```python
from build123d import *

# Parameters (mm, degrees)
SKETCH_1_W      = 44
SKETCH_1_H      = 3
SKETCH_1_H_2    = 10
EXTRUDE_1_DEPTH = 4
SKETCH_1_3_W    = 44
SKETCH_1_3_H    = 3
EXTRUDE_2_DEPTH = 30
FILLET_1_R      = 1


with BuildPart() as part:
    # Sketch 1 → Extrude 1 (new body)
    with BuildSketch(Plane.XY):
        with BuildLine():
            ThreePointArc((-22, 1), (-21.707106781, 0.292893219), (-21, 0))
            Line((-21, 0), (21, 0))
            ThreePointArc((21, 0), (21.707106781, 0.292893219), (22, 1))
            Line((22, 1), (22, 104))
            Line((22, 104), (-22, 104))
            Line((-22, 104), (-22, 1))
        make_face()
        with BuildLine():
            ThreePointArc((3.25, 7), (0, 3.75), (-3.25, 7))
            Line((-3.25, 7), (-3.25, 57))
            ThreePointArc((-3.25, 57), (0, 60.25), (3.25, 57))
            Line((3.25, 57), (3.25, 7))
        make_face(mode=Mode.SUBTRACT)
        with BuildLine():
            ThreePointArc((-15.25, 97), (-12, 100.25), (-8.75, 97))
            Line((-8.75, 97), (-8.75, 47))
            ThreePointArc((-8.75, 47), (-12, 43.75), (-15.25, 47))
            Line((-15.25, 47), (-15.25, 97))
        make_face(mode=Mode.SUBTRACT)
        with BuildLine():
            Line((8.75, 47), (8.75, 97))
            ThreePointArc((8.75, 97), (12, 100.25), (15.25, 97))
            Line((15.25, 97), (15.25, 47))
            ThreePointArc((15.25, 47), (12, 43.75), (8.75, 47))
        make_face(mode=Mode.SUBTRACT)
        with Locations((0, 105.5)):
            Rectangle(SKETCH_1_W, SKETCH_1_H)
        with Locations((0, 112)):
            Rectangle(SKETCH_1_W, SKETCH_1_H_2)
        with BuildLine():
            Line((-22, 120), (-22, 117))
            Line((-22, 117), (22, 117))
            Line((22, 117), (22, 120))
            ThreePointArc((22, 120), (21.707106781, 120.707106781), (21, 121))
            Line((21, 121), (-21, 121))
            ThreePointArc((-21, 121), (-21.707106781, 120.707106781), (-22, 120))
        make_face()
    extrude(amount=EXTRUDE_1_DEPTH)

    # Sketch 1_3 → Extrude 2 (add)
    with BuildSketch(Plane.XY):
        with Locations((0, 105.5)):
            Rectangle(SKETCH_1_3_W, SKETCH_1_3_H)
        with BuildLine():
            Line((-22, 120), (-22, 117))
            Line((-22, 117), (22, 117))
            Line((22, 117), (22, 120))
            ThreePointArc((22, 120), (21.707106781, 120.707106781), (21, 121))
            Line((21, 121), (-21, 121))
            ThreePointArc((-21, 121), (-21.707106781, 120.707106781), (-22, 120))
        make_face()
    extrude(amount=-EXTRUDE_2_DEPTH)

    # Fillet 1
    fillet_1_edges = [part.edges().sort_by_distance(p)[0] for p in [
        (-22, 105.5, -30),
        (22, 105.5, -30),
        (0, 104, -30),
        (0, 107, -30),
        (0, 121, -30),
        (21.707106781, 120.707106781, -30),
        (22, 118.5, -30),
        (0, 117, -30),
        (-22, 118.5, -30),
        (-21.707106781, 120.707106781, -30),
    ]]
    fillet(fillet_1_edges, radius=FILLET_1_R)


solid = part.part
```
The model under review builds one solid part; all positions refer to its coordinate system, in mm. A direction names the side the tool comes from. Round coordinates to 2 decimals unless told otherwise and drop trailing zeros. Loops run counter-clockwise (first coordinate to the right, second up) from the corner with the lowest first, then second, coordinate; pieces in that order, holes last. Notation, with made-up numbers: M 78.25,-2.5 L 131.25,-2.5 A17 cw 131.25,30.5 Z; hole C 3.5,87.25 d6. An arc over 180 degrees is marked long. Write item = value, one per line.
Item 1: The part is to be moulded in two halves that separate along X. For faces 1 (the cylindrical face through (0.07, 3.75, 1.97)), 2 (the cylindrical face through (-12.07, 100.25, 1.97)), 3 (the flat face through (-22, 78, 2)), 4 (the flat face through (0, 112, 0)), say which applies: released by +X, released by -X, zero draft, split by the parting line, or undercut.
Return value:
face_1 = undercut
face_2 = undercut
face_3 = released by -X
face_4 = zero draft
Item 2: Insertion check: P1, Ø13, axis at x = -0.5, y = 31, coming from the -Z side; P2, Ø4, axis at x = -4, z = -24, coming from the -Y side. Each pin has a flat end and moves straight along its axis. Give the tip position at first contact, or say it passes through.
Return value:
P1 = 0
P2 = 104
Item 3: Take a section at A-A on z = -27. Write out the cut boundary in (x, y).
Return value:
outline = M -22,104 L 22,104 L 22,107 L -22,107 Z; M -22,117 L 22,117 L 22,120 A1 ccw 21,121 L -21,121 A1 ccw -22,120 Z
Item 4: Take a section at B-B on y = 52.5. Write out the cut boundary in (x, z), then the cut area to 3 significant figures.
Return value:
outline = M -22,0 L -15.25,0 L -15.25,4 L -22,4 Z; M -8.75,0 L -3.25,0 L -3.25,4 L -8.75,4 Z; M 3.25,0 L 8.75,0 L 8.75,4 L 3.25,4 Z; M 15.25,0 L 22,0 L 22,4 L 15.25,4 Z
area = 98.0 mm2
Item 5: Take a section at C-C on x = 0. Write out the cut boundary in (y, z), then the cut area to 3 significant figures.
Return value:
outline = M 0,0 L 3.75,0 L 3.75,4 L 0,4 Z; M 60.25,0 L 104,0 L 104,-29 A1 ccw 105,-30 L 106,-30 A1 ccw 107,-29 L 107,0 L 117,0 L 117,-29 A1 ccw 118,-30 L 120,-30 A1 ccw 121,-29 L 121,4 L 60.25,4 Z
area = 467 mm2
Item 6: For line 1 (Y direction, x = 13, z = -22.5); line 2 (Z direction, x = -5.5, y = 22), list the stretches that pass through material, from the lowest coordinate up. Write a range as [from, to].
Return value:
line_1 = [104, 107], [117, 121]
line_2 = [0, 4]
Item 7: Take a section at D-D on x = -7. Write out the cut boundary in (y, z).
Return value:
outline = M 0,0 L 104,0 L 104,-29 A1 ccw 105,-30 L 106,-30 A1 ccw 107,-29 L 107,0 L 117,0 L 117,-29 A1 ccw 118,-30 L 120,-30 A1 ccw 121,-29 L 121,4 L 0,4 Z
Item 8: Machinability: for faces 5 (the cylindrical face through (-11.93, 43.75, 1.97)), 6 (the flat face through (-5, 53, 0)), 7 (the flat face through (22, 78, 1)), which of the approach directions +Z, -Z, +X, -X, +Y, -Y give a long, thin tool a straight path to every point of the face, cutting with its end or side? Answer none if there is none.
Return value:
face_5 = +Z, -Z
face_6 = -Z, +X, -X, -Y
face_7 = +Z, -Z, +X, +Y, -Y
